```python
from build123d import *

# Parameters (mm, degrees)
F2_W     = 6.975
F2_H     = 40
F2_H_2   = 6.975
F2_W_2   = 6.05
F2_R     = 2.55
F2_H_3   = 6.05
F2_W_3   = 40
F3_DEPTH = 4.2625
F4_DEPTH = 4.7625
F5_R     = 2


with BuildPart() as f3:
    # F2 (on Top) → F3 (new body)
    with BuildSketch(Plane.XY):
        with Locations((-6.5125, 30)):
            Rectangle(F2_W, F2_H)
        with Locations((-6.5125, 6.5125)):
            Rectangle(F2_W, F2_H_2)
        with Locations((0, 30)):
            Rectangle(F2_W_2, F2_H)
        with Locations((0, 20)):
            Circle(F2_R, mode=Mode.SUBTRACT)
        with Locations((0, 40)):
            Circle(F2_R, mode=Mode.SUBTRACT)
        with Locations((-6.5125, 0)):
            Rectangle(F2_W, F2_H_3)
        with Locations((6.5125, 30)):
            Rectangle(F2_W, F2_H)
        with Locations((-6.5125, -6.5125)):
            Rectangle(F2_W, F2_H_2)
        Polygon((50, 10), (10, 50), (10, 10), align=None)
        with Locations((0, -6.5125)):
            Rectangle(F2_W_2, F2_H_2)
        with Locations((30, 6.5125)):
            Rectangle(F2_W_3, F2_H_2)
        with Locations((6.5125, -6.5125)):
            Rectangle(F2_W, F2_H_2)
        with Locations((30, 0)):
            Rectangle(F2_W_3, F2_H_3)
        with Locations((20, 0)):
            Circle(F2_R, mode=Mode.SUBTRACT)
        with Locations((40, 0)):
            Circle(F2_R, mode=Mode.SUBTRACT)
        with Locations((30, -6.5125)):
            Rectangle(F2_W_3, F2_H_2)
        with Locations((6.5125, 6.5125)):
            Rectangle(F2_W, F2_H_2)
        with Locations((6.5125, 0)):
            Rectangle(F2_W, F2_H_3)
        Rectangle(F2_W_2, F2_H_3)
        Circle(F2_R, mode=Mode.SUBTRACT)
        with Locations((0, 6.5125)):
            Rectangle(F2_W_2, F2_H_2)
    extrude(amount=F3_DEPTH)

    # F2 (on Top) → F4 (join)
    with BuildSketch(Plane.XY):
        Rectangle(F2_W_2, F2_H_3)
        Circle(F2_R, mode=Mode.SUBTRACT)
        with Locations((30, 0)):
            Rectangle(F2_W_3, F2_H_3)
        with Locations((20, 0)):
            Circle(F2_R, mode=Mode.SUBTRACT)
        with Locations((40, 0)):
            Circle(F2_R, mode=Mode.SUBTRACT)
        with Locations((0, 30)):
            Rectangle(F2_W_2, F2_H)
        with Locations((0, 20)):
            Circle(F2_R, mode=Mode.SUBTRACT)
        with Locations((0, 40)):
            Circle(F2_R, mode=Mode.SUBTRACT)
    extrude(amount=F4_DEPTH)

    # F5
    f5_edges = [f3.edges().sort_by_distance(p)[0] for p in [
        (50, 10, 2.13125),
        (50, -10, 2.13125),
        (-10, -10, 2.13125),
        (-10, 50, 2.13125),
        (10, 50, 2.13125),
    ]]
    fillet(f5_edges, radius=F5_R)


solid = f3.part
```
Geometry: final body of the model. Coordinates: model frame, mm. Coordinates: 2 decimals unless noted, no trailing zeros. Loops run counter-clockwise (first coordinate to the right, second up) from the corner with the lowest first, then second, coordinate; pieces in that order, holes last. Notation, with made-up numbers: (-33, -39.75) -> (20, -39.75) arc R5 cw to (20, -34.75) -> close; hole circle Ø10 at (10.5, 81.5). An arc over 180 degrees is marked (long way). Use a Markdown table: item, result. Add a question column.
(1) Pin query (flat end, axial travel): pin 1 Ø5 at (x, y) = (20, 4.5) entering from +Z; pin 2 Ø4 at (x, y) = (37.5, 12.5) entering from +Z. Return the tip coordinate at first contact, or that it passes through.
(2) Section query B-B, the plane y = 0. State how many separate pieces and enclosed holes the cut face has, plus the area to 3 significant figures.
(3) Mould query, pull axis Y, two halves, no side actions, for faces 1 (the cylindrical face through (17.452, 0.112, 2.348)), 2 (the flat face through (1, 50, 2)), 3 (the flat face through (0, 30, 4.762)). Classes: pulls with the +Y half, pulls with the -Y half, needs draft (parallel to the pull), parting line crosses it, or undercut.
(4) Line query: line 1 along Y through (x, z) = (0, 1.4); line 2 along Z through (x, y) = (13, 26.5); line 3 along Y through (x, z) = (-2, 4.15). Output: solid intervals per line, ascending.
(5) Section query C-C, the plane z = 1.2. Return loops of the section in (x, y).
Answer:
| question | item | result |
|---|---|---|
| 1 | pin 1 | stops at z = 4.76 |
| 1 | pin 2 | stops at z = 4.26 |
| 2 | separate pieces | 4 |
| 2 | enclosed holes | 0 |
| 2 | area | 206 mm^2 |
| 3 | face 1 | undercut |
| 3 | face 2 | pulls with the +Y half |
| 3 | face 3 | needs draft |
| 4 | line 1 | y = -10 to -2.55, 2.55 to 17.45, 22.55 to 37.45, 42.55 to 50 |
| 4 | line 2 | z = 0 to 4.26 |
| 4 | line 3 | y = -10 to -1.58, 1.58 to 18.42, 21.58 to 38.42, 41.58 to 50 |
| 5 | outline | (-10, -8) arc R2 ccw to (-8, -10) -> (48, -10) arc R2 ccw to (50, -8) -> (50, 9.17) arc R2 ccw to (49.41, 10.59) -> (10.59, 49.41) arc R2 ccw to (9.17, 50) -> (-8, 50) arc R2 ccw to (-10, 48) -> close; hole circle Ø5.1 at (0, 0); hole circle Ø5.1 at (0, 20); hole circle Ø5.1 at (0, 40); hole circle Ø5.1 at (20, 0); hole circle Ø5.1 at (40, 0) |
